Read the model definition and answer for the solid it produces. Units are mm, in the model's axes. Face numbers are marked on the shaded views. A direction names the side the tool comes from. Give positions to 0.01 mm unless a question says otherwise; leave off trailing zeros. Order: outer loops, then holes, each group sorted by start corner. A loop starts at its lowest first (then second) coordinate and runs counter-clockwise, first axis right, second up. Notation, with made-up numbers: (31, -16.75) - (37, -16.75) arc R17 ccw to (37, -3.75) - close; hole circle Ø9 at (38, -35). An arc over 180 degrees is marked (long way). Write each question's results on one line, items separated by ' | '. Start each with the question number.
Q1. Find section A-A on y = 0. Give the vertices of the cut face in (x, z), and give its area (3 significant figures).
Q2. A tool of negligible diameter and unlimited length cuts with its end or side. For the marked faces 1 and 2, from which of +Z, -Z, +X, -X, +Y, -Y can it reach the whole face along a straight path? Write none if from no direction.
Q3. Flat-ended cylindrical pins translate along their axes: P1, Ø1.5, axis at y = -1.5, z = 13, coming from the +X side; P2, Ø4, axis at x = 1, z = 4, coming from the -Y side; P3, Ø1.2, axis at x = -0.5, y = -1, coming from the -Z side. Find the tip coordinate at first contact, or state that the pin passes through.
Q4. Find section C-C on z = 23.5. Give the vertices of the cut face in (x, y).
Q5. For a pull along X with two mould halves and no side action, classify the marked faces 3, 4 and 5 as +X half, -X half, draft (parallel to the pull), parting line (faces both ways), or undercut.
Q6. Find section D-D on z = 16. Give the vertices of the cut face in (x, y).
Q7. Find the intervals of material crossed by line 1 along Y through (x, z) = (0, 0.05); line 2 along Z through (x, y) = (0, 1.5); line 3 along X through (y, z) = (-0.75, 0.5), in increasing order. Write a range as from..to.
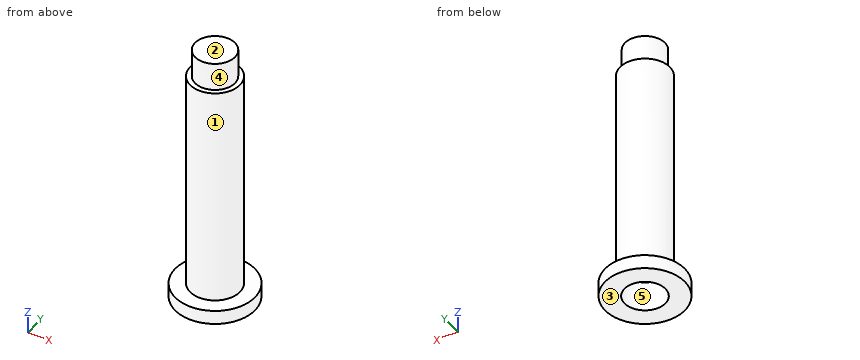
from build123d import *

# Parameters (mm, degrees)
SKETCH1_R           = 2.5
BOSS_EXTRUDE1_DEPTH = 22.25
SKETCH2_R           = 4
BOSS_EXTRUDE2_DEPTH = 1.4
SKETCH3_R           = 2.05
CUT_EXTRUDE1_DEPTH  = 3
SKETCH4_R           = 2
BOSS_EXTRUDE3_DEPTH = 2.8


with BuildPart() as part:
    # Sketch1 → Boss-Extrude1 (new body)
    with BuildSketch(Plane(origin=(0, 0, 0), x_dir=(0, 1, 0), z_dir=(0, 0, 1))):
        with Locations(Location((0, 0, 0), (0, 0, 270))):
            Circle(SKETCH1_R)
    extrude(amount=BOSS_EXTRUDE1_DEPTH)

    # Sketch2 → Boss-Extrude2 (add)
    with BuildSketch(Plane(origin=(0, 0, 0), x_dir=(1, 0, 0), z_dir=(0, 0, -1))):
        with Locations(Location((0, 0, 0), (0, 0, 180))):
            Circle(SKETCH2_R)
    extrude(amount=BOSS_EXTRUDE2_DEPTH)

    # Sketch3 → Cut-Extrude1 (cut)
    with BuildSketch(Plane(origin=(0, 0, -1.4), x_dir=(1, 0, 0), z_dir=(0, 0, -1))):
        with Locations(Location((0, 0, 0), (0, 0, 180))):
            Circle(SKETCH3_R)
    extrude(amount=-CUT_EXTRUDE1_DEPTH, mode=Mode.SUBTRACT)

    # Sketch4 → Boss-Extrude3 (add)
    with BuildSketch(Plane.XY.offset(22.25)):
        Circle(SKETCH4_R)
    extrude(amount=BOSS_EXTRUDE3_DEPTH)


solid = part.part
Working result:
1) outline: (-4, -1.4) - (-2.05, -1.4) - (-2.05, 1.6) - (2.05, 1.6) - (2.05, -1.4) - (4, -1.4) - (4, 0) - (2.5, 0) - (2.5, 22.25) - (2, 22.25) - (2, 25.05) - (-2, 25.05) - (-2, 22.25) - (-2.5, 22.25) - (-2.5, 0) - (-4, 0) - close | area: 121 mm²
2) face 1: +Z | face 2: +Z, +X, -X, +Y, -Y
3) P1: x = 2.38 | P2: y = -2.5 | P3: z = 1.6
4) outline: circle Ø4 at (0, 0)
5) face 3: draft | face 4: parting line | face 5: undercut
6) outline: circle Ø5 at (0, 0)
7) line 1: -2.5..-2.05, 2.05..2.5 | line 2: 1.6..25.05 | line 3: -2.38..-1.91, 1.91..2.38
